Read the model definition and answer for the solid it produces. Units are mm, in the model's axes. Face numbers are marked on the shaded views. A direction names the side the tool comes from. Coordinates: 2 decimals unless noted, no trailing zeros. Order: outer loops, then holes, each group sorted by start corner. A loop starts at its lowest first (then second) coordinate and runs counter-clockwise, first axis right, second up. Notation, with made-up numbers: (3, 57) -> (59, 57) arc R25 ccw to (59, 70) -> close; hole circle Ø1 at (-6, 40.25). An arc over 180 degrees is marked (long way). Use CSV: the item, a comma, the result in double quotes.
```python
from build123d import *

# Parameters (mm, degrees)
BOSS_EXTRUDE1_DEPTH = 52
SKETCH2_W           = 41
SKETCH2_H           = 23
CUT_EXTRUDE1_DEPTH  = 92
SKETCH3_W           = 10
SKETCH3_H           = 52
CUT_EXTRUDE2_DEPTH  = 9.031229
CUT_EXTRUDE3_DEPTH  = 35
SKETCH5_W           = 20
SKETCH5_H           = 38
CUT_EXTRUDE4_DEPTH  = 62
SKETCH6_W           = 9.816407164
SKETCH6_H           = 23
CUT_EXTRUDE5_DEPTH  = 11
SKETCH8_R           = 5.5
CUT_EXTRUDE6_DEPTH  = 52


with BuildPart() as part:
    # Sketch1 → Boss-Extrude1 (new body)
    with BuildSketch(Plane(origin=(0, 0, 0), x_dir=(1, 0, 0), z_dir=(0, 1, 0))):
        Polygon((0, 30.5), (0, -30.5), (28, -30.5), (28, -20.5), (77.968771248, -20.5), (110.968771248, -4.404824577), (110.968771248, 4.404824577), (77.968771248, 20.5), (28, 20.5), (28, 30.5), align=None)
    extrude(amount=BOSS_EXTRUDE1_DEPTH)

    # Sketch2 → Cut-Extrude1 (cut)
    with BuildSketch(Plane(origin=(110.968771248, 0, 0), x_dir=(0, 0, -1), z_dir=(1, 0, 0))):
        with Locations((0, 40.5)):
            Rectangle(SKETCH2_W, SKETCH2_H)
    extrude(amount=-CUT_EXTRUDE1_DEPTH, mode=Mode.SUBTRACT)

    # Sketch3 → Cut-Extrude2 (cut)
    with BuildSketch(Plane(origin=(28, 0, 0), x_dir=(0, 0, -1), z_dir=(1, 0, 0))):
        with Locations((-25.5, 26)):
            Rectangle(SKETCH3_W, SKETCH3_H)
        with Locations((25.5, 26)):
            Rectangle(SKETCH3_W, SKETCH3_H)
    extrude(amount=-CUT_EXTRUDE2_DEPTH, mode=Mode.SUBTRACT)

    # Sketch4 → Cut-Extrude3 (cut)
    with BuildSketch(Plane(origin=(0, 52, 0), x_dir=(1, 0, 0), z_dir=(0, 1, 0))):
        Polygon((120, 0), (120, 12.404317322), (98, 12.404317322), (98, -13.293630883), (120, -13.293630883), align=None)
    extrude(amount=-CUT_EXTRUDE3_DEPTH, mode=Mode.SUBTRACT)

    # Sketch5 → Cut-Extrude4 (cut)
    with BuildSketch(Plane(origin=(0, 52, 0), x_dir=(1, 0, 0), z_dir=(0, 1, 0))):
        Rectangle(SKETCH5_W, SKETCH5_H)
    extrude(amount=-CUT_EXTRUDE4_DEPTH, mode=Mode.SUBTRACT)

    # Sketch6 → Cut-Extrude5 (cut)
    with BuildSketch(Plane(origin=(0, 52, 0), x_dir=(1, 0, 0), z_dir=(0, 1, 0))):
        with Locations((14.060567666, 0)):
            Rectangle(SKETCH6_W, SKETCH6_H)
    extrude(amount=-CUT_EXTRUDE5_DEPTH, mode=Mode.SUBTRACT)

    # Sketch8 → Cut-Extrude6 (cut, through all)
    with BuildSketch(Plane.XY.offset(20.5)):
        with Locations((77.968771248, 17)):
            Circle(SKETCH8_R)
    extrude(amount=-CUT_EXTRUDE6_DEPTH, mode=Mode.SUBTRACT)


solid = part.part
```
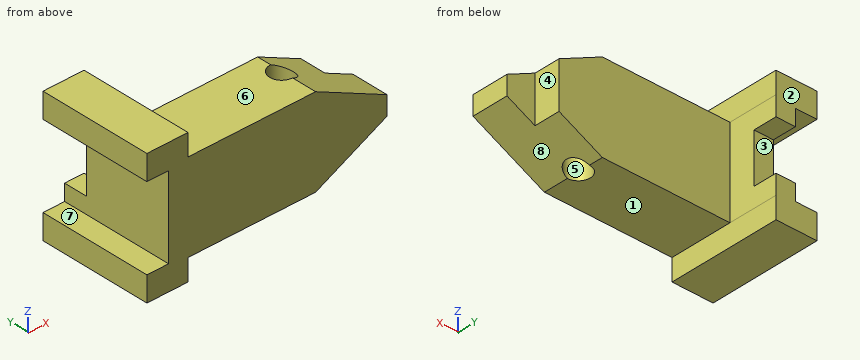
Item 1: Find section C-C, the plane x = 14. Give the vertices of the cut face in (y, z), then the cut area to 3 significant figures.
Return value:
outline,"(0, -30.5) -> (52, -30.5) -> (52, -11.5) -> (41, -11.5) -> (41, 11.5) -> (52, 11.5) -> (52, 30.5) -> (0, 30.5) -> close"
area,"2,920 mm^2"
Item 2: Straight lines are drawn through the part: line 1 along Y through (x, z) = (95, 7); line 2 along Z through (x, y) = (47.5, 26.5); line 3 along Y through (x, z) = (18, -8). For each, find the intervals that lie inside material, in ascending order.
Return value:
line 1,"y = 0 to 29"
line 2,"z = -20.5 to 20.5"
line 3,"y = 0 to 41"
Item 3: Each of these flat-tipped pins is pushed along its axis until it touches: P1, Ø4, axis at y = 45, z = -8, coming from the -X side; P2, Ø6.5, axis at x = 103, z = -4.5, coming from the +Y side; P3, Ø5, axis at y = 21.5, z = 24, coming from the +X side; P4, Ø12, axis at x = 32, z = 6.5, coming from the +Y side. Where does it stop, or does it pass through?
Return value:
P1,"passes through"
P2,"stops at y = 17"
P3,"stops at x = 18.97"
P4,"stops at y = 29"
Item 4: Find section A-A, the plane y = 43.5. Give the vertices of the cut face in (x, z).
Return value:
outline,"(0, -30.5) -> (18.97, -30.5) -> (18.97, -11.5) -> (10, -11.5) -> (10, -19) -> (0, -19) -> close; (0, 19) -> (10, 19) -> (10, 11.5) -> (18.97, 11.5) -> (18.97, 30.5) -> (0, 30.5) -> close"
Item 5: A tool of negligible diameter and unlimited length cuts with its end or side. For the marked faces 1, 2, 3 and 4, from which of +Z, -Z, +X, -X, +Y, -Y can it reach the whole face along a straight path? Write none if from no direction.
Return value:
face 1,"-Z, +X, +Y, -Y"
face 2,"+Z, -Z, +X, -X, +Y"
face 3,"+X, -X, +Y"
face 4,"+Z, -Z, +X, +Y"
Item 6: The mould has two halves that part along Z. Classify the marked faces 5, 6, 7 and 8: +Z half, -Z half, draft (parallel to the pull), parting line (faces both ways), or undercut.
Return value:
face 5,"draft"
face 6,"+Z half"
face 7,"undercut"
face 8,"-Z half"
Item 7: Find section D-D, the plane z = -16.5. Give the vertices of the cut face in (x, y).
Return value:
outline,"(10, 0) -> (86.17, 0) -> (86.17, 29) -> (18.97, 29) -> (18.97, 52) -> (10, 52) -> close; hole circle Ø11 at (77.97, 17)"
Item 8: Find section B-B, the plane z = 0. Give the vertices of the cut face in (x, y).
Return value:
outline,"(10, 0) -> (110.97, 0) -> (110.97, 17) -> (98, 17) -> (98, 29) -> (18.97, 29) -> (18.97, 41) -> (10, 41) -> close; hole circle Ø11 at (77.97, 17)"
